Study the drawing (mm; zero at the part's minimum x, y, z) and answer. A direction names the side the tool comes from. Round coordinates to 2 decimals unless told otherwise and drop trailing zeros. Write each loop counter-clockwise with the first axis right and the second up, starting at its lowest first coordinate (ties: lowest second). Pieces come first, ordered by that corner, then holes.
(1) A cutting plane is placed at C-C, the plane x = 6. Give the vertices of the cut face in (y, z).
(2) A cutting plane is placed at B-B, the plane x = 30. Give the vertices of the cut face in (y, z).
(3) Find the intervals of material crossed by probe 1 along Y at (x, z) = (30, 8.5); probe 2 along X at (y, z) = (36, 10.75); probe 3 along X at (y, z) = (17, 3.5), in increasing order.
(4) A cutting plane is placed at D-D, the plane z = 16. Give the vertices of the cut face in (x, y), and give its area (3 significant figures).
(5) A cutting plane is placed at A-A, the plane y = 55. Give the vertices of the cut face in (x, z), and give its area (3 significant figures).
(6) For the marked faces 1, 2 and 3, determine the directions among +Z, -Z, +X, -X, +Y, -Y from which every point of the face is accessible in a straight line to the end or side of a thin tool.
(7) Each of these flat-tipped pins is pushed along its axis until it touches: pin 1 Ø8 at (x, y) = (30, 55) entering from +Z; pin 2 Ø10 at (x, z) = (66.5, 9.5) entering from -Y; pin 3 Ø4 at (x, z) = (37.5, 8) entering from +Y; pin 4 Ø8 at (y, z) = (35.5, 6.5) entering from -X. Where does it stop, or does it pass through?
(8) The mould has two halves that part along Y. Classify the marked faces 4, 5 and 6: +Y half, -Y half, draft (parallel to the pull), parting line (faces both ways), or undercut.
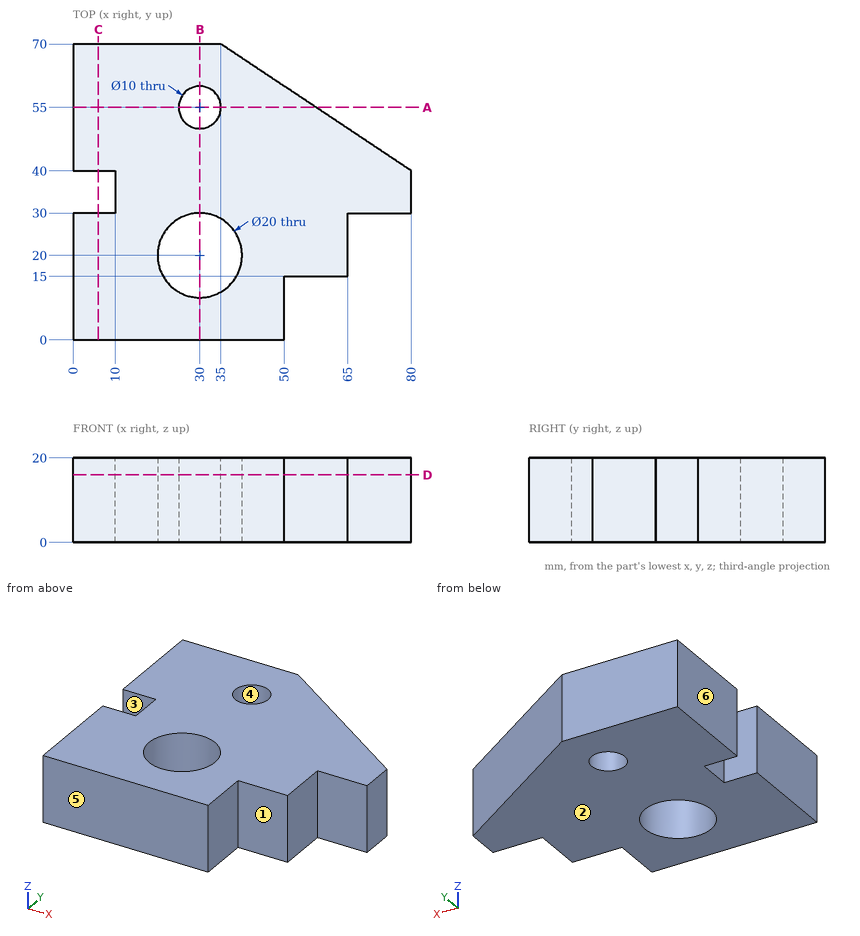
Solutions:
1. outline: (0, 0) - (30, 0) - (30, 20) - (0, 20) - close; (40, 0) - (70, 0) - (70, 20) - (40, 20) - close
2. outline: (0, 0) - (10, 0) - (10, 20) - (0, 20) - close; (30, 0) - (50, 0) - (50, 20) - (30, 20) - close; (60, 0) - (70, 0) - (70, 20) - (60, 20) - close
3. probe 1: y = 0 to 10, 30 to 50, 60 to 70
3. probe 2: x = 10 to 80
3. probe 3: x = 0 to 20.46, 39.54 to 65
4. outline: (0, 0) - (50, 0) - (50, 15) - (65, 15) - (65, 30) - (80, 30) - (80, 40) - (35, 70) - (0, 70) - (0, 40) - (10, 40) - (10, 30) - (0, 30) - close; hole circle Ø20 at (30, 20); hole circle Ø10 at (30, 55)
4. area: 3,760 mm2
5. outline: (0, 0) - (25, 0) - (25, 20) - (0, 20) - close; (35, 0) - (57.5, 0) - (57.5, 20) - (35, 20) - close
5. area: 950 mm2
6. face 1: +Z, -Z, +X, -Y
6. face 2: -Z, +X, -X, +Y, -Y
6. face 3: +Z, -Z, -X
7. pin 1: passes through
7. pin 2: stops at y = 15
7. pin 3: stops at y = 69.67
7. pin 4: stops at x = 10
8. face 4: undercut
8. face 5: -Y half
8. face 6: draft
